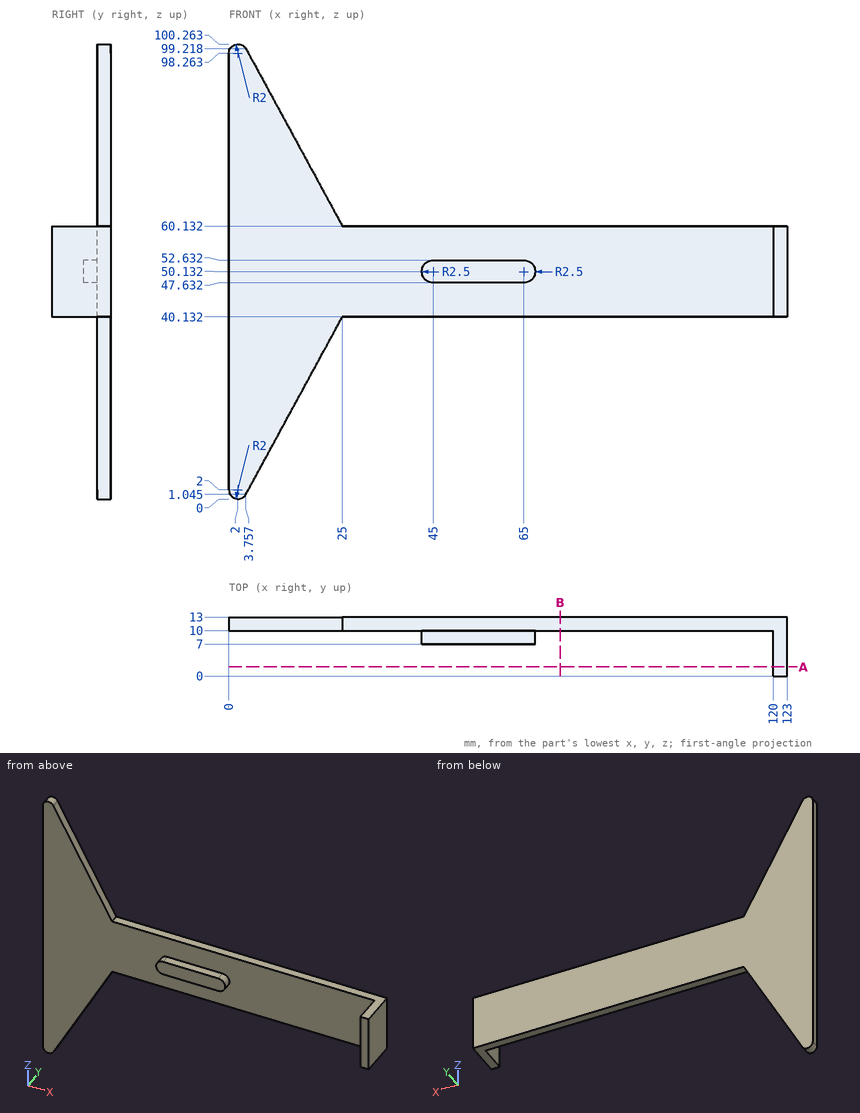
Job drawing, mm, ordinate dimensions from the low corner. One solid piece. Give positions to 0.01 mm unless a question says otherwise; leave off trailing zeros. Loops run counter-clockwise (first coordinate to the right, second up) from the corner with the lowest first, then second, coordinate; pieces in that order, holes last.
Item 1: Slice it at B-B, the plane x = 73. List the corners of the cut face in (y, z).
Answers follow:
outline: (10, 40.13) - (13, 40.13) - (13, 60.13) - (10, 60.13) - close
Item 2: Slice it at A-A, the plane y = 2. List the corners of the cut face in (x, z), and give its area (3 significant figures).
Answers follow:
outline: (120, 40.13) - (123, 40.13) - (123, 60.13) - (120, 60.13) - close
area: 60.0 mm2
Item 3: Drill centre lines: line 1 (Z direction, x = 67, y = 10.5); line 2 (X direction, y = 7.25, z = 57); line 3 (Z direction, x = 59.5, y = 8.25). Where is each one in solid material? Low to high.
Answers follow:
line 1: z = 40.13 to 60.13
line 2: x = 120 to 123
line 3: z = 47.63 to 52.63
Item 4: Flat gauge pins, fed straight in: pin 1 (4 mm diameter, centred on x = 100, y = 10, fed in from -Z); pin 2 (1 mm diameter, centred on x = 14.5, y = 10.5, fed in from +Z); pin 3 (1.5 mm diameter, centred on x = 53, y = 9, fed in from +Z); pin 4 (6.5 mm diameter, centred on x = 58, y = 3.5, fed in from +Z). Where does each tip first touch, or does it go through?
Answers follow:
pin 1: stops at z = 40.13
pin 2: stops at z = 80.37
pin 3: stops at z = 52.63
pin 4: passes through
